Geometry check sheet. Reference: the model listing, model coordinates, mm. Coordinates: 2 decimals unless noted, no trailing zeros. Write each loop counter-clockwise with the first axis right and the second up, starting at its lowest first coordinate (ties: lowest second). Pieces come first, ordered by that corner, then holes. Notation, with made-up numbers: (67.25, 20) -> (118.25, 20) arc R13 ccw to (118.25, 36) -> close; hole circle Ø6 at (57, -9.75). An arc over 180 degrees is marked (long way). Use a Markdown table: item, result.
```python
from build123d import *

# Parameters (mm, degrees)
F0_W     = 150
F0_H     = 30
F1_DEPTH = 10
F3_D     = 20
F4_SIZE  = 5


with BuildPart() as f1:
    # F0 (on Top) → F1 (new body)
    with BuildSketch(Plane.XY):
        Rectangle(F0_W, F0_H)
    extrude(amount=F1_DEPTH)

    # F3 (through all)
    with Locations(Plane.XY.offset(10)):
        with Locations((-55, 0)):
            Hole(F3_D / 2)

    # F4
    f4_edges = [f1.edges().sort_by_distance(p)[0] for p in [
        (-75, -15, 5),
        (-75, 15, 5),
    ]]
    chamfer(f4_edges, length=F4_SIZE)


solid = f1.part
```
Item 1: Thickness scan on L1, parallel to Y at x = -55, z = 3.5; L2, parallel to X at y = 7.75, z = 3.5; L3, parallel to X at y = -9.25, z = 3.75. Record the ranges inside material, lowest first. Write a range as [from, to].
Answer block:
| item | result |
|---|---|
| L1 | y = [-15, -10], [10, 15] |
| L2 | x = [-75, -61.32], [-48.68, 75] |
| L3 | x = [-75, -58.8], [-51.2, 75] |
Item 2: Mould release check, pull along X, two halves, no side actions. Record for faces 1 (the cylindrical face through (-45, 0, 5)), 2 (the flat face through (75, 0, 5)), 3 (the flat face through (-1, 0, 10)), 4 (the flat face through (-72, 13, 5)): +X half, -X half, draft (parallel to the pull), parting line (faces both ways), or undercut.
Answer block:
| item | result |
|---|---|
| face 1 | undercut |
| face 2 | +X half |
| face 3 | draft |
| face 4 | -X half |
Item 3: Section check B-B on y = 0. Record the boundary of the cut face in (x, z).
Answer block:
| item | result |
|---|---|
| outline | (-75, 0) -> (-65, 0) -> (-65, 10) -> (-75, 10) -> close; (-45, 0) -> (75, 0) -> (75, 10) -> (-45, 10) -> close |
Item 4: Section check A-A on x = -55. Record the boundary of the cut face in (y, z), then the cut area to 3 significant figures.
Answer block:
| item | result |
|---|---|
| outline | (-15, 0) -> (-10, 0) -> (-10, 10) -> (-15, 10) -> close; (10, 0) -> (15, 0) -> (15, 10) -> (10, 10) -> close |
| area | 100 mm^2 |
Item 5: Depth check by flat-ended pin: P1, Ø1, axis at x = 6, y = 6.5, coming from the -Z side. Enter the tip coordinate at first touch or a pass-through.
Answer block:
| item | result |
|---|---|
| P1 | stops at z = 0 |
Item 6: Section check C-C on z = 4. Record the boundary of the cut face in (x, y).
Answer block:
| item | result |
|---|---|
| outline | (-75, -10) -> (-70, -15) -> (75, -15) -> (75, 15) -> (-70, 15) -> (-75, 10) -> close; hole circle Ø20 at (-55, 0) |
Item 7: Section check D-D on y = 12.5. Record the boundary of the cut face in (x, z), then the cut area to 4 significant figures.
Answer block:
| item | result |
|---|---|
| outline | (-72.5, 0) -> (75, 0) -> (75, 10) -> (-72.5, 10) -> close |
| area | 1,475 mm^2 |
